Geometry check sheet. Reference: the model listing, model coordinates, mm. A direction names the side the tool comes from. Coordinates: 2 decimals unless noted, no trailing zeros. Write each loop counter-clockwise with the first axis right and the second up, starting at its lowest first coordinate (ties: lowest second). Pieces come first, ordered by that corner, then holes. Notation, with made-up numbers: (-19, 10) - (26, 10) arc R20 ccw to (26, 32) - close; hole circle Ø2 at (64, 16). An arc over 180 degrees is marked (long way). Answer as a JSON object with one key per item and string values. Group by question number.
from build123d import *

# Parameters (mm, degrees)
SKETCH1_W               = 10
SKETCH1_H               = 6
BOSS_EXTRUDE1_DEPTH     = 3.3
SKETCH2_R               = 3
BOSS_EXTRUDE2_DEPTH     = 1.2
CUT_EXTRUDE1_DEPTH      = 8.365459931
CUT_EXTRUDE1_DEPTH_BACK = 8.365459931
SKETCH3_R               = 2
CHAMFER1_SIZE           = 2


with BuildPart() as part:
    # Sketch1 → Boss-Extrude1 (new body)
    with BuildSketch(Plane(origin=(0, 0, 0), x_dir=(1, 0, 0), z_dir=(0, 1, 0))):
        Rectangle(SKETCH1_W, SKETCH1_H)
    extrude(amount=-BOSS_EXTRUDE1_DEPTH)

    # Sketch2 → Boss-Extrude2 (add)
    with BuildSketch(Plane(origin=(0, 0, 0), x_dir=(1, 0, 0), z_dir=(0, 1, 0))):
        with Locations(Location((0, 0, 0), (0, 0, 270))):
            Circle(SKETCH2_R)
    extrude(amount=BOSS_EXTRUDE2_DEPTH)

    # Sketch3 → Cut-Extrude1 (cut, two sides: drawn at the far end of the back side and taken through both)
    with BuildSketch(Plane(origin=(0, 1.2, 0), x_dir=(1, 0, 0), z_dir=(0, 1, 0)).offset(-CUT_EXTRUDE1_DEPTH_BACK)):
        with Locations(Location((0, 0, 0), (0, 0, 270))):
            Circle(SKETCH3_R)
    extrude(amount=CUT_EXTRUDE1_DEPTH + CUT_EXTRUDE1_DEPTH_BACK, mode=Mode.SUBTRACT)

    # Chamfer1
    chamfer1_edges = [part.edges().sort_by_distance(p)[0] for p in [
        (-5, -3.3, 0),
        (5, -3.3, 0),
    ]]
    chamfer(chamfer1_edges, length=CHAMFER1_SIZE)


solid = part.part
(1) Section check D-D (z = -1.3). Record the cut outline in (x, y).
(2) Section check B-B (y = -0.5). Record the cut outline in (x, z).
(3) Material ranges on L1, parallel to Z at x = 0, y = -2.1; L2, parallel to Z at x = 1, y = -2.8, recorded low to high. Write a range as [from, to].
(4) Draft check along Z on faces 3 (the face through (0, -2, -3)), 4 (the face through (-2, -1, 0)), 5 (the face through (0, -2, 3)). Enter one of: +Z half, -Z half, draft (parallel to the pull), parting line (faces both ways), or undercut.
(5) Section check A-A (z = 0). Record the cut outline in (x, y).
(6) Gauge pin test, flat end, axial feed: pin 1 (3.5 mm diameter, centred on x = 0, z = 0, fed in from -Y). Record the tip position at first contact, or that the pin passes through.
(7) Set-up check for faces 1 (the face through (0.9, 0.59, 2.86)), 2 (the face through (4, -2.3, 0)): record each of +Z, -Z, +X, -X, +Y, -Y from which the full face is reachable in a straight line by a thin tool's end or side.
(8) Section check C-C (x = -2.75). Record the cut outline in (y, z).
Conclusion:
{
 "1": {"outline": "(-5, -1.3) - (-3, -3.3) - (-1.52, -3.3) - (-1.52, 1.2) - (-2.7, 1.2) - (-2.7, 0) - (-5, 0) - close; (1.52, -3.3) - (3, -3.3) - (5, -1.3) - (5, 0) - (2.7, 0) - (2.7, 1.2) - (1.52, 1.2) - close"},
 "2": {"outline": "(-5, -3) - (5, -3) - (5, 3) - (-5, 3) - close; hole circle Ø4 at (0, 0)"},
 "3": {"L1": "z = [-3, -2], [2, 3]", "L2": "z = [-3, -1.73], [1.73, 3]"},
 "4": {"face 3": "-Z half", "face 4": "undercut", "face 5": "+Z half"},
 "5": {"outline": "(-5, -1.3) - (-3, -3.3) - (-2, -3.3) - (-2, 1.2) - (-3, 1.2) - (-3, 0) - (-5, 0) - close; (2, -3.3) - (3, -3.3) - (5, -1.3) - (5, 0) - (3, 0) - (3, 1.2) - (2, 1.2) - close"},
 "6": {"pin 1": "passes through"},
 "7": {"face 1": "+Y", "face 2": "+Z, -Z, +X, -Y"},
 "8": {"outline": "(-3.3, -3) - (0, -3) - (0, -1.2) - (1.2, -1.2) - (1.2, 1.2) - (0, 1.2) - (0, 3) - (-3.3, 3) - close"}
}
